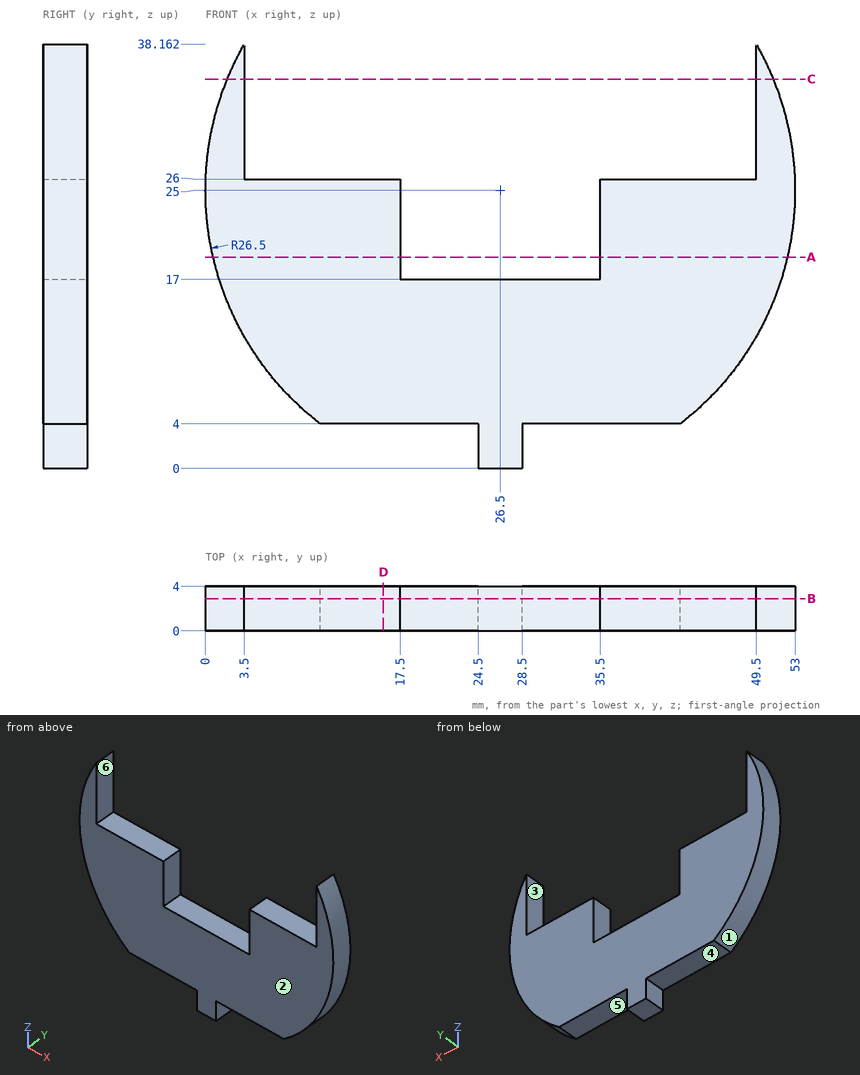
Source: three-view drawing plus pictorial views. Frame: mm from the lowest corner of the part. A direction names the side the tool comes from. Round coordinates to 2 decimals unless told otherwise and drop trailing zeros. Loops run counter-clockwise (first coordinate to the right, second up) from the corner with the lowest first, then second, coordinate; pieces in that order, holes last. Notation, with made-up numbers: (-23.75, 2) - (16.25, 2) arc R11 cw to (16.25, 19) - close; hole circle Ø11 at (48.5, -5.5). An arc over 180 degrees is marked (long way). Write each question's results on one line, items separated by ' | '. Start each with the question number.
1) Cut plane C-C on z = 35. Return loops of the section in (x, y).
2) Mould query, pull axis X, two halves, no side actions, for the marked faces 1, 2 and 3. Classes: released by +X, released by -X, zero draft, split by the parting line, or undercut.
3) Cut plane B-B on y = 2.9. Return loops of the section in (x, z).
4) First-contact query: P1, Ø1.5, axis at x = 21, y = 2.5, coming from the +Z side; P2, Ø1.2, axis at y = 1.5, z = 33, coming from the +X side (1 decimal); P3, Ø2, axis at y = 2.5, z = 2, coming from the +X side. Flat tips, straight axial feed; report the tip coordinate or a pass-through.
5) Cut plane A-A on z = 19. Return loops of the section in (x, y).
6) Line query: probe 1 along Z at (x, y) = (34, 2.2); probe 2 along Z at (x, y) = (36, 0.5); probe 3 along X at (y, z) = (2.85, 2). Output: solid intervals per line, ascending. Write a range as [from, to].
7) Access query for the marked faces 4, 5 and 6. Directions: +Z, -Z, +X, -X, +Y, -Y. A direction counts if a zero-diameter tool reaches every point of the face in a straight line with its end or side. Return the directions, or none.
8) Cut plane D-D on x = 16. Return loops of the section in (y, z).
Verdict:
1) outline: (1.96, 0) - (3.5, 0) - (3.5, 4) - (1.96, 4) - close; (49.5, 0) - (51.04, 0) - (51.04, 4) - (49.5, 4) - close
2) face 1: released by -X | face 2: zero draft | face 3: undercut
3) outline: (3.5, 26) - (3.5, 38.16) arc R26.5 ccw to (10.34, 4) - (24.5, 4) - (24.5, 0) - (28.5, 0) - (28.5, 4) - (42.66, 4) arc R26.5 ccw to (49.5, 38.16) - (49.5, 26) - (35.5, 26) - (35.5, 17) - (17.5, 17) - (17.5, 26) - close
4) P1: stops at z = 17 | P2: stops at x = 51.9 | P3: stops at x = 28.5
5) outline: (0.69, 0) - (17.5, 0) - (17.5, 4) - (0.69, 4) - close; (35.5, 0) - (52.31, 0) - (52.31, 4) - (35.5, 4) - close
6) probe 1: z = [4, 17] | probe 2: z = [4, 26] | probe 3: x = [24.5, 28.5]
7) face 4: -Z, -X, +Y, -Y | face 5: -Z, +X, +Y, -Y | face 6: +Z, +Y, -Y
8) outline: (0, 4) - (4, 4) - (4, 26) - (0, 26) - close
